Build history of the part. All positions in model axes, mm. Give positions to 0.01 mm unless a question says otherwise; leave off trailing zeros. Order: outer loops, then holes, each group sorted by start corner. A loop starts at its lowest first (then second) coordinate and runs counter-clockwise, first axis right, second up. Notation, with made-up numbers: M 1.25,36.25 L 10.25,36.25 A15 cw 10.25,49.25 Z; hole C 30.5,-3 d9. An arc over 180 degrees is marked long. Use CSV: the item, a comma, the result in double quotes. Start each with the question number.
Item 1: Band-saw the part on B-B on y = -8. Write the cut outline in (x, z), plus the area to 3 significant figures.
Item 2: Band-saw the part on A-A on z = 18. Write the cut outline in (x, y).
Item 3: Wall check: line 1 along Z through (x, y) = (-4, -43); line 2 along X through (y, z) = (-20.5, 13); line 3 along Z through (x, y) = (-12.5, -69). Give the ranges that are in metal, low to high.
Item 4: Pin check, flat tips, straight feed: P1, Ø10, axis at x = -12.5, y = -35, coming from the +Z side; P2, Ø1, axis at x = -12.5, z = 21, coming from the +Y side; P3, Ø1, axis at x = -7, y = -86.5, coming from the +Z side; P4, Ø6, axis at x = -25.5, y = -72.5, coming from the +Z side. Stop position of each tip, or through.
Item 5: Two-plate mould, pull along Y, no slides. Class faces 1 (the flat face through (0, -14, 21)), 2 (the cylindrical face through (-15.211, -86.346, 35.855)): pulls with the +Y half, pulls with the -Y half, needs draft (parallel to the pull), parting line crosses it, or undercut.
from build123d import *

# Parameters (mm, degrees)
F1_DEPTH  = 100
F8_R      = 0.25
F9_DEPTH  = 76.7908446712
F3_R      = 5
F3_R_2    = 4.5
F3_R_3    = 4
F3_R_4    = 3.5
F3_R_5    = 3
F3_R_6    = 2.5
F3_R_7    = 2
F3_R_8    = 1.5
F3_R_9    = 1
F10_DEPTH = 42.4274068712


with BuildPart() as f1:
    # F0 (on Front) → F1 (new body)
    with BuildSketch(Plane.XZ):
        Polygon((0, 0), (0, 42.4264068712), (-30, 30), (-30, 0), align=None)
    extrude(amount=F1_DEPTH)

    # F8 (on line) → F9 (cut, through all)
    with BuildSketch(Plane(origin=(13.0839062865, 5.4195314327, 5.4195314327), x_dir=(-0.3302007759, 0.9339488311, -0.1367736397), z_dir=(0.8628562095, 0.3574067443, 0.3574067443))):
        with Locations((-13.2744047348, 39.1968889463)):
            Circle(F8_R)
        with Locations((-24.9487651235, 39.1968889463)):
            Circle(F8_R)
        with Locations((-35.6891766811, 39.1968889463)):
            Circle(F8_R)
        with Locations((-45.4956394075, 39.1968889463)):
            Circle(F8_R)
        with Locations((-54.3681533029, 39.1968889463)):
            Circle(F8_R)
        with Locations((-62.3067183672, 39.1968889463)):
            Circle(F8_R)
        with Locations((-69.3113346005, 39.1968889463)):
            Circle(F8_R)
        with Locations((-75.3820020026, 39.1968889463)):
            Circle(F8_R)
        with Locations((-80.5187205736, 39.1968889463)):
            Circle(F8_R)
    extrude(amount=-F9_DEPTH, mode=Mode.SUBTRACT)

    # F3 (on plane+point) → F10 (cut, through all)
    with BuildSketch(Plane.XY.offset(42.4264068712)):
        with Locations((0, -8)):
            Circle(F3_R)
        with Locations((0, -20.5)):
            Circle(F3_R_2)
        with Locations((0, -32)):
            Circle(F3_R_3)
        with Locations((0, -42.5)):
            Circle(F3_R_4)
        with Locations((0, -52)):
            Circle(F3_R_5)
        with Locations((0, -60.5)):
            Circle(F3_R_6)
        with Locations((0, -68)):
            Circle(F3_R_7)
        with Locations((0, -74.5)):
            Circle(F3_R_8)
        with Locations((0, -80)):
            Circle(F3_R_9)
    extrude(amount=-F10_DEPTH, mode=Mode.SUBTRACT)


solid = f1.part
Model answer:
1,outline,"M -30,0 L -5,0 L -5,40.36 L -30,30 Z"
1,area,"879 mm^2"
2,outline,"M -30,-100 L 0,-100 L 0,-81 A1 cw 0,-79 L 0,-76 A1.5 cw 0,-73 L 0,-70 A2 cw 0,-66 L 0,-63 A2.5 cw 0,-58 L 0,-55 A3 cw 0,-49 L 0,-46 A3.5 cw 0,-39 L 0,-36 A4 cw 0,-28 L 0,-25 A4.5 cw 0,-16 L 0,-13 A5 cw 0,-3 L 0,0 L -30,0 Z"
3,line 1,"z = 0 to 40.77"
3,line 2,"x = -30 to -4.5"
3,line 3,"z = 0 to 37.25"
4,P1,"stops at z = 39.32"
4,P2,"stops at y = 0"
4,P3,"stops at z = 39.73"
4,P4,"stops at z = 33.11"
5,face 1,"needs draft"
5,face 2,"undercut"
